Source: CAD feature listing. Evaluate the final solid. Frame: model axes, mm. A direction names the side the tool comes from. Round coordinates to 2 decimals unless told otherwise and drop trailing zeros. Write each loop counter-clockwise with the first axis right and the second up, starting at its lowest first coordinate (ties: lowest second). Pieces come first, ordered by that corner, then holes.
```python
from build123d import *

# Parameters (mm, degrees)
F0_W     = 25
F0_H     = 30
F1_DEPTH = 6.5
F2_R     = 1.5
F3_DEPTH = 6.501
F4_W     = 1
F4_H     = 6.1
F5_DEPTH = 0.9
F6_SIZE  = 10
F7_R     = 10


with BuildPart() as f1:
    # F0 (on Top) → F1 (new body)
    with BuildSketch(Plane.XY):
        Rectangle(F0_W, F0_H)
    extrude(amount=F1_DEPTH)

    # F2 (on face) → F3 (cut, through all)
    with BuildSketch(Plane.XY.offset(6.5)):
        with Locations((-2, -12)):
            Circle(F2_R)
        with Locations((4.5, -1.5)):
            Circle(F2_R)
        with Locations((4.5, 8.5)):
            Circle(F2_R)
    extrude(amount=-F3_DEPTH, mode=Mode.SUBTRACT)

    # F4 (on face) → F5 (cut)
    with BuildSketch(Plane(origin=(0, 0, 0), x_dir=(1, 0, 0), z_dir=(0, 0, -1))):
        with Locations((11.6, 6.95)):
            Rectangle(F4_W, F4_H)
        with Locations((9.6, 6.95)):
            Rectangle(F4_W, F4_H)
        with Locations((7.6, 6.95)):
            Rectangle(F4_W, F4_H)
        with Locations((5.6, 6.95)):
            Rectangle(F4_W, F4_H)
        with Locations((3.6, 6.95)):
            Rectangle(F4_W, F4_H)
        with Locations((1.6, 6.95)):
            Rectangle(F4_W, F4_H)
        with Locations((-0.4, 6.95)):
            Rectangle(F4_W, F4_H)
        with Locations((-2.4, 6.95)):
            Rectangle(F4_W, F4_H)
        with Locations((-4.4, 6.95)):
            Rectangle(F4_W, F4_H)
        with Locations((-6.4, 6.95)):
            Rectangle(F4_W, F4_H)
        with Locations((-8.4, 6.95)):
            Rectangle(F4_W, F4_H)
        with Locations((-10.4, 6.95)):
            Rectangle(F4_W, F4_H)
        with Locations((-12.4, 6.95)):
            Rectangle(F4_W, F4_H)
    extrude(amount=-F5_DEPTH, mode=Mode.SUBTRACT)

    # F6
    f6_edges = [f1.edges().sort_by_distance(p)[0] for p in [
        (-12.5, 15, 3.25),
    ]]
    chamfer(f6_edges, length=F6_SIZE)

    # F7
    f7_edges = [f1.edges().sort_by_distance(p)[0] for p in [
        (-12.5, 5, 3.25),
        (-2.5, 15, 3.25),
        (12.5, 15, 3.25),
    ]]
    fillet(f7_edges, radius=F7_R)


solid = f1.part
```
Q1. Section query A-A, the plane y = -1.5. Output: boundary loops of the cut face in (x, z).
Q2. Mould query, pull axis Y, two halves, no side actions, for faces 1 (the face through (9.6, -3.9, 0.4)), 2 (the face through (0, 0, 0)). Classes: pulls with the +Y half, pulls with the -Y half, needs draft (parallel to the pull), parting line crosses it, or undercut.
Q3. Section query C-C, the plane z = 3. Output: boundary loops of the cut face in (x, y).
Q4. Section query D-D, the plane x = -7.25. Output: boundary loops of the cut face in (y, z), and give its area (3 significant figures).
Q5. Section query B-B, the plane x = 4.5. Output: boundary loops of the cut face in (y, z), and give its area (3 significant figures).
Q6. Line query: line 1 (Y direction, x = 4.5, z = 3.5); line 2 (Y direction, x = -0.25, z = 0.5); line 3 (Z direction, x = 8, y = -6.5). Output: solid intervals per line, ascending.
Q7. Set-up query: faces 3 (the face through (5.886, -2.075, 3.296)), 4 (the face through (-10.4, -10, 0.4)). Return all of +Z, -Z, +X, -X, +Y, -Y with unobstructed straight access to the full face (end or side cutting, diameter ignored); none if empty.
Q8. Pin query (flat end, axial travel): P1, Ø0.7, axis at y = -8, z = 0.5, coming from the -X side; P2, Ø2, axis at y = 8, z = 3, coming from the +X side; P3, Ø1.5, axis at x = -3, z = 4.5, coming from the +Y side. Return the tip coordinate at first contact, or that it passes through.
Filled in:
1. outline: (-12.5, 0) - (3, 0) - (3, 6.5) - (-12.5, 6.5) - close; (6, 0) - (12.5, 0) - (12.5, 6.5) - (6, 6.5) - close
2. face 1: undercut
2. face 2: needs draft
3. outline: (-12.5, -15) - (12.5, -15) - (12.5, 5) arc R10 ccw to (2.5, 15) - (1.64, 15) arc R10 ccw to (-5.43, 12.07) - (-9.57, 7.93) arc R10 ccw to (-12.5, 0.86) - close; hole circle Ø3 at (-2, -12); hole circle Ø3 at (4.5, -1.5); hole circle Ø3 at (4.5, 8.5)
4. outline: (-15, 0) - (10.25, 0) - (10.25, 6.5) - (-15, 6.5) - close
4. area: 164 mm2
5. outline: (-15, 0) - (-3, 0) - (-3, 6.5) - (-15, 6.5) - close; (0, 0) - (7, 0) - (7, 6.5) - (0, 6.5) - close; (10, 0) - (14.8, 0) - (14.8, 6.5) - (10, 6.5) - close
5. area: 155 mm2
6. line 1: y = -15 to -3, 0 to 7, 10 to 14.8
6. line 2: y = -15 to -10, -3.9 to 14.82
6. line 3: z = 0.9 to 6.5
7. face 3: +Z, -Z
7. face 4: -Z
8. P1: stops at x = -11.9
8. P2: stops at x = 12.3
8. P3: stops at y = 14.21
